The model under review builds one solid part; all positions refer to its coordinate system, in mm. A direction names the side the tool comes from. Round coordinates to 2 decimals unless told otherwise and drop trailing zeros. Loops run counter-clockwise (first coordinate to the right, second up) from the corner with the lowest first, then second, coordinate; pieces in that order, holes last. Notation, with made-up numbers: (48, 85) - (56, 85) arc R23 cw to (56, 124) - close; hole circle Ø9 at (87.25, 58.25). An arc over 180 degrees is marked (long way). Answer as CSV lines item,"result".
from build123d import *

# Parameters (mm, degrees)
BOSS_EXTRUDE1_DEPTH = 5
SKETCH2_R           = 1.5
CUT_EXTRUDE1_DEPTH  = 5
SKETCH5_W           = 20
SKETCH5_H           = 5
BOSS_EXTRUDE3_DEPTH = 2
CUT_EXTRUDE2_REACH  = 24.535
SKETCH6_R           = 1.75


with BuildPart() as part:
    # Sketch1 → Boss-Extrude1 (new body)
    with BuildSketch(Plane(origin=(0, 0, 0), x_dir=(1, 0, 0), z_dir=(0, 1, 0))):
        Polygon((0, 0), (0, 3), (10.567063084, 9.100896716), (10.567063084, 3), (20, 3), (20, 0), align=None)
    extrude(amount=BOSS_EXTRUDE1_DEPTH)

    # Sketch2 → Cut-Extrude1 (cut)
    with BuildSketch(Plane(origin=(-1.299038106, 0, -2.25), x_dir=(-0.8660254037844397, 0, 0.49999999999999806), z_dir=(-0.49999999999999806, 0, -0.8660254037844397))):
        with Locations((-7.5, 2.5)):
            Circle(SKETCH2_R)
    extrude(amount=-CUT_EXTRUDE1_DEPTH, mode=Mode.SUBTRACT)

    # Sketch5 → Boss-Extrude3 (add)
    with BuildSketch(Plane.XY):
        with Locations((10, 2.5)):
            Rectangle(SKETCH5_W, SKETCH5_H)
    extrude(amount=BOSS_EXTRUDE3_DEPTH)

    # Cut-Extrude2: up to this face of the body (flat: up to its plane)
    cut_extrude2_end = Plane(part.part.faces().sort_by_distance((0, 2.5, -0.5))[0])
    # Sketch6 → Cut-Extrude2 (cut, up to the picked face)
    with BuildSketch(Plane(origin=(20, 0, 0), x_dir=(0, 0, -1), z_dir=(1, 0, 0)), mode=Mode.PRIVATE) as cut_extrude2_sk1:
        with Locations((0.25, 2.5)):
            Circle(SKETCH6_R)
    cut_extrude2_tool1 = split(extrude(cut_extrude2_sk1.sketch, amount=-CUT_EXTRUDE2_REACH, mode=Mode.PRIVATE), bisect_by=cut_extrude2_end, keep=Keep.BOTH, mode=Mode.PRIVATE)
    add(cut_extrude2_tool1.solids().sort_by(Axis((20, 2.5, -0.25), (-1, 0, 0)))[0], mode=Mode.SUBTRACT)


solid = part.part
1. Take a section at D-D (y = 3.6). State the section outline as (x, z) points.
Numbers:
outline,"(0, -3) - (4.31, -5.49) - (6.55, -1.61) - (0, -1.61) - close; (0, 1.11) - (20, 1.11) - (20, 2) - (0, 2) - close; (6.08, -6.51) - (10.57, -9.1) - (10.57, -3) - (20, -3) - (20, -1.61) - (7.59, -1.61) - (8.58, -2.18) - close"
2. Wall thickness on probe 1 along Y at (x, z) = (14, -0.25); probe 2 along Z at (x, y) = (17, 2.7); probe 3 along X at (y, z) = (1.2, -3.75): over which ranges is each line inside the solid? List them lowest first.
Numbers:
probe 1,"y = 0 to 0.75, 4.25 to 5"
probe 2,"z = -3 to -1.99, 1.49 to 2"
probe 3,"x = 1.3 to 5.63, 7.36 to 10.57"
3. Take a section at B-B (y = 2.5). State the section outline as (x, z) points, plus the area to 3 significant figures.
Numbers:
outline,"(0, -3) - (3.9, -5.25) - (5.77, -2) - (0, -2) - close; (0, 1.5) - (20, 1.5) - (20, 2) - (0, 2) - close; (6.5, -6.75) - (10.57, -9.1) - (10.57, -3) - (20, -3) - (20, -2) - (8.27, -2) - (9, -2.42) - close"
area,"48.6 mm²"
4. Draft analysis for pull direction Z (two halves, no side actions). For faces 1 (the face through (5.2, 0.8, -6)), 2 (the face through (8.49, 2.19, -2.13)), 3 (the face through (10, 3, 2)), state which applies: +Z half, -Z half, draft (parallel to the pull), parting line (faces both ways), or undercut.
Numbers:
face 1,"-Z half"
face 2,"undercut"
face 3,"+Z half"
5. Take a section at A-A (z = -0.25). State the section outline as (x, y) points.
Numbers:
outline,"(0, 0) - (20, 0) - (20, 0.75) - (0, 0.75) - close; (0, 4.25) - (20, 4.25) - (20, 5) - (0, 5) - close"
6. Clearance check with flat-ended pins moving along their axes: pin 1 (1 mm diameter, centred on y = 1.5, z = -4.5, fed in from +X); pin 2 (1 mm diameter, centred on x = 4.5, z = 0.5, fed in from -Y); pin 3 (1 mm diameter, centred on x = 16.5, y = 3, fed in from -Z). State where each tip first meets the part, or that it passes through.
Numbers:
pin 1,"stops at x = 10.57"
pin 2,"stops at y = 0"
pin 3,"stops at z = -3"
7. Take a section at C-C (x = 17.75). State the section outline as (y, z) points.
Numbers:
outline,"(0, -3) - (5, -3) - (5, 2) - (0, 2) - close; hole circle Ø3.5 at (2.5, -0.25)"
8. Tool access review of faces 4 (the face through (10, 0, -2)), 5 (the face through (10.567, 2, -6)): name each direction out of +Z, -Z, +X, -X, +Y, -Y from which nothing blocks a thin tool from reaching the whole face with its end or side.
Numbers:
face 4,"+Z, -Z, +X, -X, -Y"
face 5,"-Z, +X, +Y, -Y"
